Geometry check sheet. Reference: drawing and pictorial views, mm from the part's lowest x, y, z. A direction names the side the tool comes from. Round coordinates to 2 decimals unless told otherwise and drop trailing zeros. Write each loop counter-clockwise with the first axis right and the second up, starting at its lowest first coordinate (ties: lowest second). Pieces come first, ordered by that corner, then holes. Notation, with made-up numbers: (35.25, 80) - (73.25, 80) arc R29 cw to (73.25, 110) - close; hole circle Ø3 at (-39.5, 15). An arc over 180 degrees is marked (long way). Use one line per item in the form item = value. Start each with the question number.
1) Section check D-D (x = 9). Record the boundary of the cut face in (y, z).
2) Section check C-C (y = 5). Record the boundary of the cut face in (x, z), then the cut area to 3 significant figures.
3) Set-up check for the marked faces 1 and 2: record each of +Z, -Z, +X, -X, +Y, -Y from which the full face is reachable in a straight line by a thin tool's end or side.
4) Section check B-B (x = 5). Record the boundary of the cut face in (y, z).
5) Section check A-A (z = 3.75). Record the boundary of the cut face in (x, y), then the cut area to 3 significant figures.
6) Scan lines: probe 1 along Y at (x, z) = (5, 5); probe 2 along Y at (x, z) = (5, 12.25); probe 3 along X at (y, z) = (5, 3.25). Record each from-to range of solid material in increasing order.
7) Draft check along X on the marked faces 3, 4 and 5. Enter one of: +X half, -X half, draft (parallel to the pull), parting line (faces both ways), or undercut.
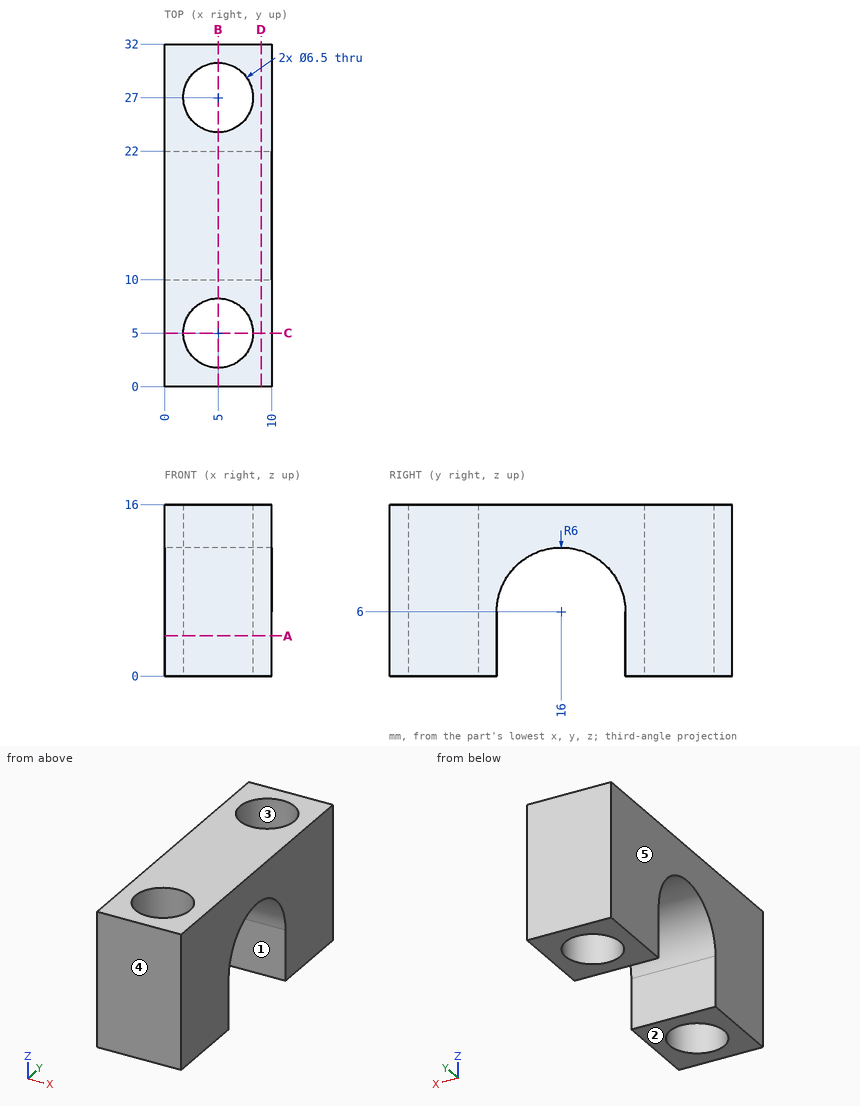
Results are:
q1.outline = (0, 0) - (10, 0) - (10, 6) arc R6 cw to (22, 6) - (22, 0) - (32, 0) - (32, 16) - (0, 16) - close
q2.outline = (0, 0) - (1.75, 0) - (1.75, 16) - (0, 16) - close; (8.25, 0) - (10, 0) - (10, 16) - (8.25, 16) - close
q2.area = 56.0 mm²
q3.face_1 = -Z, +X, -X
q3.face_2 = -Z, +X, -X, +Y, -Y
q4.outline = (0, 0) - (1.75, 0) - (1.75, 16) - (0, 16) - close; (8.25, 0) - (10, 0) - (10, 6) arc R6 cw to (22, 6) - (22, 0) - (23.75, 0) - (23.75, 16) - (8.25, 16) - close; (30.25, 0) - (32, 0) - (32, 16) - (30.25, 16) - close
q5.outline = (0, 0) - (10, 0) - (10, 10) - (0, 10) - close; (0, 22) - (10, 22) - (10, 32) - (0, 32) - close; hole circle Ø6.5 at (5, 5); hole circle Ø6.5 at (5, 27)
q5.area = 134 mm²
q6.probe_1 = 0 to 1.75, 8.25 to 10, 22 to 23.75, 30.25 to 32
q6.probe_2 = 0 to 1.75, 8.25 to 23.75, 30.25 to 32
q6.probe_3 = 0 to 1.75, 8.25 to 10
q7.face_3 = undercut
q7.face_4 = draft
q7.face_5 = -X half
